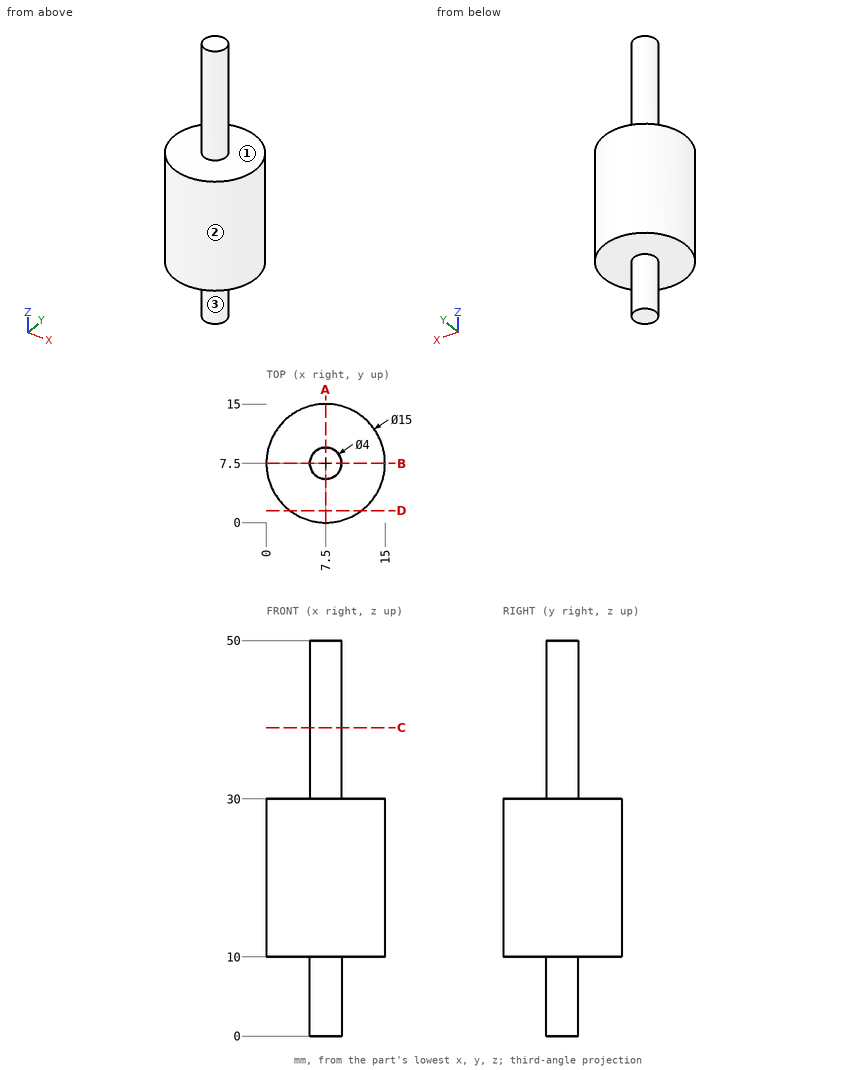
Study the drawing (mm; zero at the part's minimum x, y, z) and answer. A direction names the side the tool comes from. Give positions to 0.01 mm unless a question says otherwise; leave off trailing zeros. Write each loop counter-clockwise with the first axis right and the second up, starting at its lowest first coordinate (ties: lowest second). Pieces come first, ordered by that corner, then holes. Notation, with made-up numbers: (-38.75, 12.5) - (-9.75, 12.5) arc R36 ccw to (-9.75, 46.5) - close; hole circle Ø1 at (-1.75, 49.25). An arc over 180 degrees is marked (long way). Use a Markdown table: item, result.
1. Section C-C on z = 39 is taken. Write down the section's boundary in (x, y).
Values follow:
| item | result |
|---|---|
| outline | circle Ø4 at (7.5, 7.5) |
2. Each of these flat-tipped pins is pushed along its axis until it touches: P1, Ø2, axis at x = 11.5, y = 9.5, coming from the +Z side; P2, Ø5, axis at x = 6, z = 29, coming from the +Y side; P3, Ø3, axis at x = 2, z = 26, coming from the +Y side; P4, Ø3, axis at x = 5, z = 22, coming from the -Y side. Where does it stop, or does it pass through?
Values follow:
| item | result |
|---|---|
| P1 | stops at z = 30 |
| P2 | stops at y = 15 |
| P3 | stops at y = 13.84 |
| P4 | stops at y = 0.07 |
3. Find the intervals of material crossed by probe 1 along Z at (x, y) = (9.5, 0.75); probe 2 along Y at (x, z) = (12, 21); probe 3 along X at (y, z) = (4.25, 18), in increasing order. Write a range as from..to.
Values follow:
| item | result |
|---|---|
| probe 1 | z = 10..30 |
| probe 2 | y = 1.5..13.5 |
| probe 3 | x = 0.74..14.26 |
4. A tool of negligible diameter and unlimited length cuts with its end or side. For the marked faces 1, 2 and 3, from which of +Z, -Z, +X, -X, +Y, -Y can it reach the whole face along a straight path? Write none if from no direction.
Values follow:
| item | result |
|---|---|
| face 1 | +Z |
| face 2 | +Z, -Z |
| face 3 | -Z |
5. Section A-A on x = 7.5 is taken. Write down the section's boundary in (y, z).
Values follow:
| item | result |
|---|---|
| outline | (0, 10) - (5.5, 10) - (5.5, 0) - (9.5, 0) - (9.5, 10) - (15, 10) - (15, 30) - (9.5, 30) - (9.5, 50) - (5.5, 50) - (5.5, 30) - (0, 30) - close |
6. Section D-D on y = 1.5 is taken. Write down the section's boundary in (x, z).
Values follow:
| item | result |
|---|---|
| outline | (3, 10) - (12, 10) - (12, 30) - (3, 30) - close |
